```python
from build123d import *

# Parameters (mm, degrees)
SKETCH1_W               = 170
SKETCH1_H               = 70
BOSS_EXTRUDE1_DEPTH     = 30
FILLET1_R               = 10
SKETCH2_W               = 45
SKETCH2_H               = 40
SKETCH2_W_2             = 50
SKETCH2_H_2             = 10
SKETCH2_H_3             = 5
CUT_EXTRUDE1_DEPTH      = 20
SKETCH3_W               = 10
SKETCH3_H               = 10
BOSS_EXTRUDE2_DEPTH     = 10
SKETCH4_W               = 30
SKETCH4_H               = 10
BOSS_EXTRUDE3_DEPTH     = 3
SKETCH5_W               = 30
SKETCH5_H               = 30
BOSS_EXTRUDE4_DEPTH     = 10
FILLET2_R               = 2
SKETCH6_W               = 15
SKETCH6_H               = 15
CUT_EXTRUDE2_DEPTH      = 10
SKETCH7_W               = 10
SKETCH7_H               = 10
BOSS_EXTRUDE5_DEPTH     = 7
CUT_EXTRUDE3_DEPTH      = 7
CUT_EXTRUDE3_DEPTH_BACK = 13
SKETCH8_R               = 2
SKETCH9_W               = 60
SKETCH9_H               = 70
CUT_EXTRUDE4_DEPTH      = 2


with BuildPart() as part:
    # Sketch1 → Boss-Extrude1 (new body)
    with BuildSketch(Plane(origin=(0, 0, 0), x_dir=(1, 0, 0), z_dir=(0, 1, 0))):
        Rectangle(SKETCH1_W, SKETCH1_H)
    extrude(amount=BOSS_EXTRUDE1_DEPTH)

    # Fillet1
    fillet1_edges = [part.edges().sort_by_distance(p)[0] for p in [
        (-85, 30, 0),
        (0, 30, 35),
        (85, 30, 0),
        (0, 0, 35),
        (-85, 0, 0),
        (0, 0, -35),
        (85, 0, 0),
        (85, 15, 35),
        (-85, 15, 35),
        (-85, 15, -35),
        (85, 15, -35),
        (0, 30, -35),
    ]]
    fillet(fillet1_edges, radius=FILLET1_R)

    # Sketch2 → Cut-Extrude1 (cut)
    with BuildSketch(Plane(origin=(0, 30, 0), x_dir=(1, 0, 0), z_dir=(0, 1, 0))):
        with Locations((-47.5, 0)):
            Rectangle(SKETCH2_W, SKETCH2_H)
        Rectangle(SKETCH2_W_2, SKETCH2_H)
        with Locations((47.5, 0)):
            Rectangle(SKETCH2_W, SKETCH2_H)
        with Locations((0, 30)):
            Rectangle(SKETCH2_W_2, SKETCH2_H_2)
        with Locations((0, 22.5)):
            Rectangle(SKETCH2_W_2, SKETCH2_H_3)
        with Locations((0, -30)):
            Rectangle(SKETCH2_W_2, SKETCH2_H_2)
        with Locations((0, -22.5)):
            Rectangle(SKETCH2_W_2, SKETCH2_H_3)
    extrude(amount=-CUT_EXTRUDE1_DEPTH, mode=Mode.SUBTRACT)

    # Sketch3 → Boss-Extrude2 (add)
    with BuildSketch(Plane(origin=(0, 10, 0), x_dir=(1, 0, 0), z_dir=(0, 1, 0))):
        with Locations((-30, 15)):
            Rectangle(SKETCH3_W, SKETCH3_H)
        with Locations((30, 15)):
            Rectangle(SKETCH3_W, SKETCH3_H)
        with Locations((30, -15)):
            Rectangle(SKETCH3_W, SKETCH3_H)
        with Locations((-30, -15)):
            Rectangle(SKETCH3_W, SKETCH3_H)
    extrude(amount=BOSS_EXTRUDE2_DEPTH)

    # Sketch4 → Boss-Extrude3 (add)
    with BuildSketch(Plane.XY.offset(35)):
        Polygon((-40, 30), (-68.080792204, 30), (-70, 30), (-70, 0), (-40, 0), align=None)
        with Locations((55, 15)):
            Rectangle(SKETCH4_W, SKETCH4_H)
        with Locations((55, 25)):
            Rectangle(SKETCH4_W, SKETCH4_H)
        with Locations((55, 5)):
            Rectangle(SKETCH4_W, SKETCH4_H)
    extrude(amount=BOSS_EXTRUDE3_DEPTH)

    # Sketch5 → Boss-Extrude4 (add)
    with BuildSketch(Plane(origin=(0, 0, 35), x_dir=(-1, 0, 0), z_dir=(0, 0, -1))):
        with Locations((-55, 15)):
            Rectangle(SKETCH5_W, SKETCH5_H)
        with Locations((55, 15)):
            Rectangle(SKETCH5_W, SKETCH5_H)
    extrude(amount=BOSS_EXTRUDE4_DEPTH)

    # Fillet2
    fillet2_edges = [part.edges().sort_by_distance(p)[0] for p in [
        (-70, 15, 38),
        (-55, 0, 38),
        (-40, 15, 38),
        (-55, 30, 38),
        (40, 15, 38),
        (55, 30, 38),
        (55, 0, 38),
        (70, 15, 38),
    ]]
    fillet(fillet2_edges, radius=FILLET2_R)

    # Sketch6 → Cut-Extrude2 (cut)
    with BuildSketch(Plane.XY.offset(38)):
        with Locations((-55, 16)):
            Rectangle(SKETCH6_W, SKETCH6_H)
        with Locations((55, 16)):
            Rectangle(SKETCH6_W, SKETCH6_H)
    extrude(amount=-CUT_EXTRUDE2_DEPTH, mode=Mode.SUBTRACT)

    # Sketch7 → Boss-Extrude5 (add)
    with BuildSketch(Plane.XY.offset(28)):
        with Locations((-55, 16)):
            Rectangle(SKETCH7_W, SKETCH7_H)
        with Locations((55, 16)):
            Rectangle(SKETCH7_W, SKETCH7_H)
    extrude(amount=BOSS_EXTRUDE5_DEPTH)

    # Sketch8 → Cut-Extrude3 (cut, two sides: drawn at the far end of the back side and taken through both)
    with BuildSketch(Plane.XY.offset(28).offset(-CUT_EXTRUDE3_DEPTH_BACK)):
        with Locations(Location((49.5, 21.5, 0), (0, 0, 180))):
            Circle(SKETCH8_R)
        with Locations(Location((49.5, 10.5, 0), (0, 0, 180))):
            Circle(SKETCH8_R)
        with Locations(Location((60.5, 21.5, 0), (0, 0, 180))):
            Circle(SKETCH8_R)
        with Locations(Location((60.5, 10.5, 0), (0, 0, 194.477512186))):
            Circle(SKETCH8_R)
        with Locations(Location((-60.5, 10.5, 0), (0, 0, 180))):
            Circle(SKETCH8_R)
        with Locations(Location((-49.5, 10.5, 0), (0, 0, 165.522487814))):
            Circle(SKETCH8_R)
        with Locations(Location((-60.5, 21.5, 0), (0, 0, 180))):
            Circle(SKETCH8_R)
        with Locations(Location((-49.5, 21.5, 0), (0, 0, 180))):
            Circle(SKETCH8_R)
    extrude(amount=CUT_EXTRUDE3_DEPTH + CUT_EXTRUDE3_DEPTH_BACK, mode=Mode.SUBTRACT)

    # Sketch9 → Cut-Extrude4 (cut)
    with BuildSketch(Plane.XZ):
        Rectangle(SKETCH9_W, SKETCH9_H)
    extrude(amount=-CUT_EXTRUDE4_DEPTH, mode=Mode.SUBTRACT)


solid = part.part
```
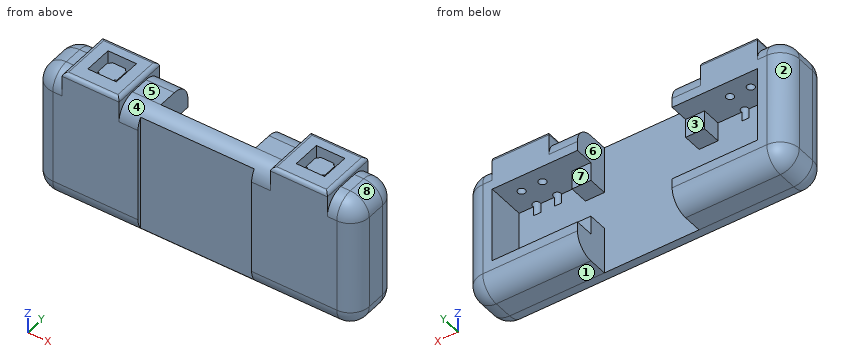
Can you work these out from the model? Positions are in its coordinate system, mm. Face numbers are marked on the shaded views. A direction names the side the tool comes from. Coordinates: 2 decimals unless noted, no trailing zeros. Loops run counter-clockwise (first coordinate to the right, second up) from the corner with the lowest first, then second, coordinate; pieces in that order, holes last. Notation, with made-up numbers: (25, 57.5) -> (65, 57.5) arc R23 ccw to (65, 76.5) -> close; hole circle Ø9 at (-16, 36). An arc over 180 degrees is marked (long way). Put each result on its own line as item: value. Start each with the question number.
Q1. For the marked faces 4, 5, 6, 7 and 8, which set-ups out of +Z, -Z, +X, -X, +Y, -Y let a thin tool reach every point of the face, with its end or its side?
Q2. Thinking about a two-plate mould opening in X: for the marked faces 1, 2 and 3, which applies, pulls with the +X half, pulls with the -X half, needs draft (parallel to the pull), parting line crosses it, or undercut?
Q3. I want a section at D-D (z = 4). Write out the boundary of the cut face in (x, y).
Q4. I want a section at B-B (z = -13.5). Write out the boundary of the cut face in (x, y).
Q5. I want a section at A-A (x = -72). Write out the boundary of the cut face in (y, z), plus the area to 3 significant figures.
Q6. I'm going to push flat-ended pins straight in: P1, Ø0.6, axis at x = 48.5, y = 22.5, coming from the +Z side; P2, Ø1.2, axis at x = -60.5, y = 18.5, coming from the +Z side; P3, Ø10, axis at x = -13.5, z = -12, coming from the +Y side. Where does each tip first touch, or does it pass through?
Q7. If I drill on line 1 (X direction, y = 10.5, z = -25.5); line 2 (X direction, y = 10.5, z = 30.5); line 3 (Z direction, x = -30.5, y = 19.5), over which ranges is the centre line in solid material (lowest first)? Write a range as [from, to].
Taken from the geometry:
1. face 4: +Z, -Y
1. face 5: +Z, +Y, -Y
1. face 6: +Z, -Z, +Y
1. face 7: +Y
1. face 8: +Z, +X, +Y, -Y
2. face 1: needs draft
2. face 2: pulls with the -X half
2. face 3: undercut
3. outline: (-85, 10) arc R10 ccw to (-75, 0) -> (-30, 0) -> (-30, 2) -> (30, 2) -> (30, 0) -> (75, 0) arc R10 ccw to (85, 10) -> (85, 20) arc R10 ccw to (75, 30) -> (70, 30) -> (70, 10) -> (-70, 10) -> (-70, 30) -> (-75, 30) arc R10 ccw to (-85, 20) -> close
4. outline: (-85, 10) arc R10 ccw to (-75, 0) -> (-30, 0) -> (-30, 2) -> (30, 2) -> (30, 0) -> (75, 0) arc R10 ccw to (85, 10) -> (85, 20) arc R10 ccw to (75, 30) -> (70, 30) -> (70, 10) -> (35, 10) -> (35, 20) -> (25, 20) -> (25, 10) -> (-25, 10) -> (-25, 20) -> (-35, 20) -> (-35, 10) -> (-70, 10) -> (-70, 30) -> (-75, 30) arc R10 ccw to (-85, 20) -> close
5. outline: (0, -25) arc R10 ccw to (10, -35) -> (20, -35) arc R10 ccw to (30, -25) -> (30, 25) arc R10 ccw to (20, 35) -> (10, 35) arc R10 ccw to (0, 25) -> close
5. area: 2,010 mm2
6. P1: stops at z = -20
6. P2: stops at z = 35
6. P3: stops at y = 10
7. line 1: x = [-84.99, -25], [25, 84.99]
7. line 2: x = [-83.35, -62.5], [-47.5, -25], [25, 47.5], [62.5, 83.35]
7. line 3: z = [-35, -10], [10, 35]
